Check sheet for the modelled part. Datum: model origin and axes. Units: mm. Round coordinates to 2 decimals unless told otherwise and drop trailing zeros. Write each loop counter-clockwise with the first axis right and the second up, starting at its lowest first coordinate (ties: lowest second). Pieces come first, ordered by that corner, then holes.
Item 1: Depth check by flat-ended pin: pin 1 (1 mm diameter, centred on y = 1, z = 15.5, fed in from -X). Enter the tip coordinate at first touch or a pass-through.
Item 2: Section check A-A, the plane z = 19. Record the cut outline in (x, y) (3 decimals).
Item 3: Material ranges on line 1 along Y through (x, z) = (0.1, 3.25); line 2 along Z through (x, y) = (1.5, 0.25), recorded low to high.
from build123d import *

# Parameters (mm, degrees)
F0_R     = 1.905
F1_DEPTH = 25.4
F2_SIZE  = 0.762
F3_DEPTH = 7.62
F4_DEPTH = 3.81


with BuildPart() as f1:
    # F0 (on Top) → F1 (new body)
    with BuildSketch(Plane.XY):
        Circle(F0_R)
    extrude(amount=F1_DEPTH)

    # F2
    f2_edges = [f1.edges().sort_by_distance(p)[0] for p in [
        (-1.905, 0, 0),
    ]]
    chamfer(f2_edges, length=F2_SIZE)

    # F3 (cut): a face of the model
    f3_faces = [f1.faces().sort_by_distance(p)[0] for p in [
        (0, 0, 25.4),
    ]]
    extrude(f3_faces, amount=-F3_DEPTH, mode=Mode.SUBTRACT)

    # F4 (add): a face of the model
    f4_faces = [f1.faces().sort_by_distance(p)[0] for p in [
        (0, 0, 17.78),
    ]]
    extrude(f4_faces, amount=F4_DEPTH)


solid = f1.part
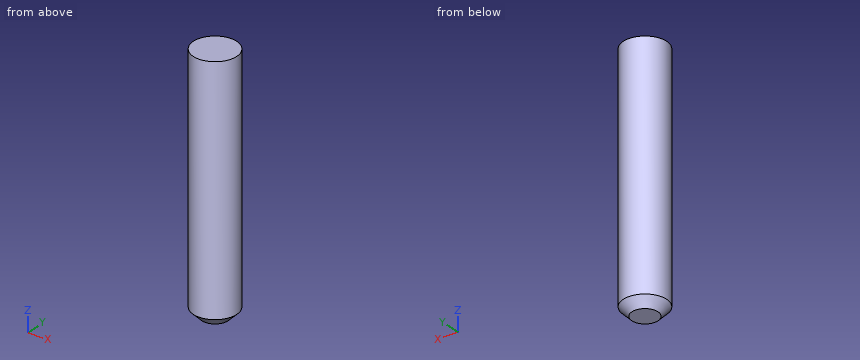
Values found:
1. pin 1: stops at x = -1.84
2. outline: circle Ø3.81 at (0, 0)
3. line 1: y = -1.9 to 1.9
3. line 2: z = 0.38 to 21.59
